Part model, mm, in its own coordinate system. A direction names the side the tool comes from. Round coordinates to 2 decimals unless told otherwise and drop trailing zeros. Loops run counter-clockwise (first coordinate to the right, second up) from the corner with the lowest first, then second, coordinate; pieces in that order, holes last. Notation, with made-up numbers: M -17.75,62 L 38.25,62 A4 ccw 38.25,66 Z; hole C 77.5,44.5 d6. An arc over 180 degrees is marked long. Put each result on its own line as item: value. Start each with the question number.
1) Probe line 1 along Y through (x, z) = (0, 3) (3 decimals); line 2 along X through (y, z) = (-2.5, 13.5); line 3 along X through (y, z) = (41, 14.75). List the from-to ranges inside material, lowest first.
2) Which spindle directions (+Z, -Z, +X, -X, +Y, -Y) get a long thin tool onto all of the face, cutting with end or side? Do faces 1 (the cylindrical face through (3.597, -84.924, 13.605)), 2 (the cylindrical face through (1.955, -0.616, 6.91)), 3 (the flat face through (-67, -53, 21)), 4 (the flat face through (-10, 80, 6)), 5 (the flat face through (1, 2, 4)). Say none if no direction does.
3) Drop flat-ended pins along their axis: pin 1 Ø2 at (y, z) = (-29.5, 7) entering from -X; pin 2 Ø1 at (y, z) = (-12.5, 11) entering from -X; pin 3 Ø3 at (x, y) = (-49, 68) entering from -Z; pin 4 Ø2.5 at (x, y) = (-38.65, 55.46) entering from -Z. Give the stop position or say it passes through.
4) Slice it at A-A on y = 0. Give the cut face in (x, z), then the cut area to 3 significant figures.
```python
from build123d import *

# Parameters (mm, degrees)
F2_R       = 2.05
F3_DEPTH   = 20
F4_W       = 20
F4_H       = 25
F5_DEPTH   = 25
F6_R       = 1.93
F7_DEPTH   = 5.8
F8_R       = 2.605
F9_DEPTH   = 25
F10_R      = 4.35
F10_R_2    = 1.65
F11_DEPTH  = 4
F11_FACE_R = 1.65
F13_DEPTH  = 25
F14_ANGLE  = -90
F15_ANGLE  = -270


with BuildPart() as f1:
    # F0 (on Front) → F1 (revolve)
    with BuildSketch(Plane.XZ):
        Polygon((-90, 0), (0, 0), (0, 10), (-85, 6), (-85, 21), (-90, 21), align=None)
    revolve(axis=Axis((0, 0, -12.121966), (0, 0, -1)))

    # F2 (on face) → F3 (cut)
    with BuildSketch(Plane(origin=(0, 0, 0), x_dir=(1, 0, 0), z_dir=(0, 0, -1))):
        Circle(F2_R)
    extrude(amount=-F3_DEPTH, mode=Mode.SUBTRACT)

    # F4 (on face) → F5 (cut)
    with BuildSketch(Plane(origin=(0, 0, 0), x_dir=(1, 0, 0), z_dir=(0, 0, -1))):
        with Locations((0, -77.625006)):
            Rectangle(F4_W, F4_H)
    extrude(amount=-F5_DEPTH, mode=Mode.SUBTRACT)

    # F6 (on face) → F7 (cut)
    with BuildSketch(Plane(origin=(0, 0, 0), x_dir=(1, 0, 0), z_dir=(0, 0, -1))):
        with Locations((-49.477956, -67.757965)):
            Circle(F6_R)
        with Locations((-50.155689, -45.322918)):
            Circle(F6_R)
        with Locations((-60.987717, -57.61691)):
            Circle(F6_R)
        with Locations((-38.645928, -55.463973)):
            Circle(F6_R)
    extrude(amount=-F7_DEPTH, mode=Mode.SUBTRACT)

    # F8 (on face) → F9 (cut)
    with BuildSketch(Plane(origin=(0, 0, 0), x_dir=(1, 0, 0), z_dir=(0, 0, -1))):
        with Locations((0, -17.655)):
            Circle(F8_R)
    extrude(amount=-F9_DEPTH, mode=Mode.SUBTRACT)

    # F10 (on face) → F11 (cut)
    with BuildSketch(Plane(origin=(0, 0, 0), x_dir=(1, 0, 0), z_dir=(0, 0, -1))):
        Circle(F10_R)
        with Locations((0, -8.56)):
            Circle(F10_R_2)
        with Locations((0, 8.56)):
            Circle(F10_R_2)
    extrude(amount=-F11_DEPTH, mode=Mode.SUBTRACT)

    # F11_face (on face) → F13 (cut)
    with BuildSketch(Plane(origin=(0, -8.56, 4), x_dir=(1, 0, 0), z_dir=(0, 0, -1))):
        Circle(F11_FACE_R)
        with Locations((0, -17.12)):
            Circle(F11_FACE_R)
    extrude(amount=-F13_DEPTH, mode=Mode.SUBTRACT)


with BuildPart() as f1_1:
    # F14: moved
    add(f1.part.rotate(Axis((-0.498306, 0, 0), (1, 0, 0)), F14_ANGLE))


with BuildPart() as f1_2:
    # F15: moved
    add(f1_1.part.rotate(Axis((-0.498306, 0, 0), (1, 0, 0)), F15_ANGLE))


solid = f1_2.part
```
Recorded:
1. line 1: y = -90 to -10.21, -6.91 to -4.35, 4.35 to 6.91, 10.21 to 15.05, 20.26 to 65.125
1. line 2: x = -89.97 to -84.96, 84.96 to 89.97
1. line 3: x = -80.12 to -74.46, 74.46 to 80.12
2. face 1: +Z
2. face 2: +Z, -Z
2. face 3: +Z, +X, -X, +Y, -Y
2. face 4: +Z, -Z, +Y
2. face 5: -Z
3. pin 1: stops at x = -85.37
3. pin 2: stops at x = -89.2
3. pin 3: stops at z = 0
3. pin 4: stops at z = 5.8
4. outline: M -90,0 L -4.35,0 L -4.35,4 L -2.05,4 L -2.05,9.9 L -85,6 L -85,21 L -90,21 Z; M 2.05,4 L 4.35,4 L 4.35,0 L 90,0 L 90,21 L 85,21 L 85,6 L 2.05,9.9 Z
4. area: 1,510 mm2
